```python
from build123d import *

# Parameters (mm, degrees)
F0_W     = 388
F0_H     = 100
F0_R     = 2
F1_DEPTH = 10
F2_R     = 3.1
F3_DEPTH = 10
F4_R     = 2
F5_DEPTH = 10


with BuildPart() as f1:
    # F0 (on Front) → F1 (new body)
    with BuildSketch(Plane.XZ):
        Rectangle(F0_W, F0_H)
        with Locations((-134, -45)):
            Circle(F0_R, mode=Mode.SUBTRACT)
        with Locations((-84, -45)):
            Circle(F0_R, mode=Mode.SUBTRACT)
        with Locations((-84, -10)):
            Circle(F0_R, mode=Mode.SUBTRACT)
        with Locations((94, -45)):
            Circle(F0_R, mode=Mode.SUBTRACT)
        with Locations((144, -45)):
            Circle(F0_R, mode=Mode.SUBTRACT)
        with Locations((16, -10)):
            Circle(F0_R, mode=Mode.SUBTRACT)
        with Locations((116, -10)):
            Circle(F0_R, mode=Mode.SUBTRACT)
    extrude(amount=F1_DEPTH)

    # F2 (on face) → F3 (cut)
    with BuildSketch(Plane.XZ.offset(10)):
        with Locations((-6, 25)):
            Circle(F2_R)
        with Locations((94, 25)):
            Circle(F2_R)
        with Locations((-106, 25)):
            Circle(F2_R)
    extrude(amount=-F3_DEPTH, mode=Mode.SUBTRACT)

    # F4 (on face) → F5 (cut)
    with BuildSketch(Plane(origin=(-194, 0, 0), x_dir=(0, -1, 0), z_dir=(-1, 0, 0))):
        with Locations((5, -30)):
            Circle(F4_R)
        with Locations((5, 30)):
            Circle(F4_R)
    extrude(amount=-F5_DEPTH, mode=Mode.SUBTRACT)


solid = f1.part
```
Work out the finished part from the listing and answer in its coordinate system (mm). Give positions to 0.01 mm unless a question says otherwise; leave off trailing zeros.
1. Straight lines are drawn through the part: L1, parallel to Z at x = 16, y = -5.5; L2, parallel to Z at x = -134, y = -3.25. For each, find the intervals that lie inside material, in ascending order.
Result sheet:
L1: z = -50 to -12, -8 to 50
L2: z = -50 to -47, -43 to 50
2. The mould has two halves that part along Z. Classify faces 1 (the flat face through (-3, -5, -50)), 2 (the flat face through (194, -5, -1)), 3 (the cylindrical face through (96.957, -5.07, 25.931)), 4 (the flat face through (-3, -5, 50)): released by +Z, released by -Z, zero draft, split by the parting line, or undercut.
Result sheet:
face 1: released by -Z
face 2: zero draft
face 3: undercut
face 4: released by +Z
3. This flat-tipped pin is pushed along its axis until it touches: P1, Ø3, axis at y = -5, z = 30, coming from the -X side. Where does it stop, or does it pass through?
Result sheet:
P1: stops at x = -184
